Work out the finished part from the listing and answer in its coordinate system (mm). Coordinates: 2 decimals unless noted, no trailing zeros. Write each loop counter-clockwise with the first axis right and the second up, starting at its lowest first coordinate (ties: lowest second). Pieces come first, ordered by that corner, then holes. Notation, with made-up numbers: M 17.5,-5.5 L 37.5,-5.5 A29 cw 37.5,27.5 Z; hole C 12.25,-38.5 d6. An arc over 180 degrees is marked long. Answer as CSV lines item,"result". Start each with the question number.
(1) Find the intervals of material crossed by L1, parallel to Z at x = 60, y = 2; L2, parallel to X at y = 0.7, z = -75; L3, parallel to Z at x = 8.5, y = 1.8, in increasing order. Write a range as [from, to].
(2) A cutting plane is placed at B-B on x = 4. Give the vertices of the cut face in (y, z).
(3) A cutting plane is placed at A-A on y = 2.4. Give the vertices of the cut face in (x, z), then the cut area to 3 significant figures.
(4) Flat-ended cylindrical pins translate along their axes: P1, Ø2.5, axis at x = 60, z = -75, coming from the -Y side; P2, Ø0.9, axis at y = 2, z = 66, coming from the +X side; P3, Ø0.9, axis at y = 1.5, z = 64.5, coming from the -X side; P4, Ø0.9, axis at x = -4, y = 1.5, coming from the -Z side. Find the tip coordinate at first contact, or state that the pin passes through.
from build123d import *

# Parameters (mm, degrees)
SKETCH1_W           = 180
SKETCH1_H           = 180
BOSS_EXTRUDE1_DEPTH = 3
SKETCH2_W           = 15
SKETCH2_H           = 75
CUT_EXTRUDE1_DEPTH  = 3
SKETCH3_R           = 1.5
CUT_EXTRUDE2_DEPTH  = 3
SKETCH4_W           = 20
SKETCH4_H           = 4
CUT_EXTRUDE3_DEPTH  = 10


with BuildPart() as part:
    # Sketch1 → Boss-Extrude1 (new body)
    with BuildSketch(Plane(origin=(0, 0, 0), x_dir=(1, 0, 0), z_dir=(0, 1, 0))):
        Rectangle(SKETCH1_W, SKETCH1_H)
    extrude(amount=BOSS_EXTRUDE1_DEPTH)

    # Sketch2 → Cut-Extrude1 (cut)
    with BuildSketch(Plane(origin=(0, 3, 0), x_dir=(1, 0, 0), z_dir=(0, 1, 0))):
        with Locations((-82.5, -47.5)):
            Rectangle(SKETCH2_W, SKETCH2_H)
        with Locations((82.5, -47.5)):
            Rectangle(SKETCH2_W, SKETCH2_H)
    extrude(amount=-CUT_EXTRUDE1_DEPTH, mode=Mode.SUBTRACT)

    # Sketch3 → Cut-Extrude2 (cut)
    with BuildSketch(Plane(origin=(0, 3, 0), x_dir=(1, 0, 0), z_dir=(0, 1, 0))):
        with Locations(Location((-60, -80, 0), (0, 0, 270))):
            Circle(SKETCH3_R)
        with Locations(Location((60, -80, 0), (0, 0, 90))):
            Circle(SKETCH3_R)
        with Locations(Location((-60, 75, 0), (0, 0, 270))):
            Circle(SKETCH3_R)
        with Locations(Location((60, 75, 0), (0, 0, 90))):
            Circle(SKETCH3_R)
    extrude(amount=-CUT_EXTRUDE2_DEPTH, mode=Mode.SUBTRACT)

    # Sketch4 → Cut-Extrude3 (cut)
    with BuildSketch(Plane(origin=(0, 3, 0), x_dir=(1, 0, 0), z_dir=(0, 1, 0))):
        with Locations((0, 88)):
            Rectangle(SKETCH4_W, SKETCH4_H)
    extrude(amount=-CUT_EXTRUDE3_DEPTH, mode=Mode.SUBTRACT)


solid = part.part
Here are the results:
1,L1,"z = [-90, -76.5], [-73.5, 78.5], [81.5, 90]"
1,L2,"x = [-90, -61.5], [-58.5, 58.5], [61.5, 90]"
1,L3,"z = [-86, 90]"
2,outline,"M 0,-86 L 3,-86 L 3,90 L 0,90 Z"
3,outline,"M -90,-90 L -10,-90 L -10,-86 L 10,-86 L 10,-90 L 90,-90 L 90,10 L 75,10 L 75,85 L 90,85 L 90,90 L -90,90 L -90,85 L -75,85 L -75,10 L -90,10 Z; hole C -60,-75 d3; hole C -60,80 d3; hole C 60,-75 d3; hole C 60,80 d3"
3,area,"30,000 mm^2"
4,P1,"passes through"
4,P2,"stops at x = 75"
4,P3,"stops at x = -75"
4,P4,"stops at z = -86"
